```python
from build123d import *

# Parameters (mm, degrees)
BOSS_EXTRU_1_DEPTH      = 10
BOSS_EXTRU_2_DEPTH      = 48
BOSS_EXTRU_3_DEPTH      = 2
CHANFREIN1_SIZE         = 6
ENL_V_MAT_EXTRU_1_REACH = 148.244
ESQUISSE5_R             = 1.75
ESQUISSE6_R             = 3.5
ENL_V_MAT_EXTRU_2_DEPTH = 4
CHANFREIN2_SIZE         = 7.5
ESQUISSE7_R             = 1.25
ENL_V_MAT_EXTRU_3_DEPTH = 10


with BuildPart() as part:
    # Esquisse1 → Boss.-Extru.1 (new body)
    with BuildSketch(Plane.XY):
        with BuildLine():
            Line((-40.181760398, -97.007350914), (-47.835429046, -115.484941564))
            ThreePointArc((-47.835429046, -115.484941564), (-24.386290252, -122.59816005), (0, -125))
            Line((0, -125), (0, -105))
            ThreePointArc((0, -105), (-20.484483812, -102.982454442), (-40.181760398, -97.007350914))
        make_face()
    extrude(amount=BOSS_EXTRU_1_DEPTH)

    # Esquisse2 → Boss.-Extru.2 (add)
    with BuildSketch(Plane.XY.offset(10)):
        with BuildLine():
            Line((-32.925344295, -102.858746361), (-38.108037379, -119.049474955))
            ThreePointArc((-38.108037379, -119.049474955), (-24.386290252, -122.59816005), (-10.351025939, -124.570687812))
            Line((-10.351025939, -124.570687812), (-8.943286411, -107.62907427))
            ThreePointArc((-8.943286411, -107.62907427), (-21.069754778, -105.924810284), (-32.925344295, -102.858746361))
        make_face()
    extrude(amount=BOSS_EXTRU_2_DEPTH)

    # Esquisse4 → Boss.-Extru.3 (add)
    with BuildSketch(Plane.XY.offset(58)):
        with BuildLine():
            Line((-39.413172773, -123.12671677), (-10.705530953, -128.837021766))
            Line((-10.705530953, -128.837021766), (-8.943286411, -107.62907427))
            ThreePointArc((-8.943286411, -107.62907427), (-21.069754778, -105.924810284), (-32.925344295, -102.858746361))
            Line((-32.925344295, -102.858746361), (-39.413172773, -123.12671677))
        make_face()
    extrude(amount=BOSS_EXTRU_3_DEPTH)

    # Chanfrein1
    # the kernel refuses this chamfer: 6 mm, written as the material it adds along each edge
    with BuildSketch(Plane(origin=(0, 0, 58), x_dir=(-0.3048642990280114, -0.9523957996432781, 0), z_dir=(-0.9523957996432781, 0.3048642990280114, 0))) as chanfrein1_piece_1_section:
        Polygon((125 + CHANFREIN1_SIZE, 0), (125, -CHANFREIN1_SIZE), (125, 0), align=None)
    chanfrein1_piece_1 = revolve(axis=Axis((0, 0, 58), (0, 0, 1)), revolution_arc=13, mode=Mode.PRIVATE)
    chanfrein1_piece_1 = split(chanfrein1_piece_1, bisect_by=Plane(origin=(-25.059351863, -125.981869268, 58), z_dir=(0.19509032201612828, 0.9807852804032304, 0)), keep=Keep.TOP, mode=Mode.PRIVATE)
    add(chanfrein1_piece_1)

    # Esquisse5 → Enlèv. mat.-Extru.1 (cut, up to next)
    with BuildSketch(Plane.XY.offset(10), mode=Mode.PRIVATE) as enl_v_mat_extru_1_sk1:
        with Locations((-4.765565521, -114.901215769)):
            Circle(ESQUISSE5_R)
    enl_v_mat_extru_1_tool1 = extrude(enl_v_mat_extru_1_sk1.sketch, amount=-ENL_V_MAT_EXTRU_1_REACH, mode=Mode.PRIVATE) & part.part
    # Esquisse5 → Enlèv. mat.-Extru.1 (cut, up to next)
    with BuildSketch(Plane.XY.offset(10), mode=Mode.PRIVATE) as enl_v_mat_extru_1_sk2:
        with Locations((-39.567983188, -107.978584481)):
            Circle(ESQUISSE5_R)
    enl_v_mat_extru_1_tool2 = extrude(enl_v_mat_extru_1_sk2.sketch, amount=-ENL_V_MAT_EXTRU_1_REACH, mode=Mode.PRIVATE) & part.part
    add(enl_v_mat_extru_1_tool1.solids().sort_by_distance((-4.765566, -114.901216, 10))[0], mode=Mode.SUBTRACT)
    add(enl_v_mat_extru_1_tool2.solids().sort_by_distance((-39.567983, -107.978584, 10))[0], mode=Mode.SUBTRACT)

    # Esquisse6 → Enlèv. mat.-Extru.2 (cut)
    with BuildSketch(Plane.XY.offset(10)):
        with Locations((-39.567983188, -107.978584481)):
            Circle(ESQUISSE6_R)
        with Locations((-4.765565521, -114.901215769)):
            Circle(ESQUISSE6_R)
    extrude(amount=-ENL_V_MAT_EXTRU_2_DEPTH, mode=Mode.SUBTRACT)

    # Chanfrein2
    # the kernel refuses this chamfer: 7.5 mm, written as the material it takes off along each edge
    with BuildSketch(Plane(origin=(-8.943286411, -107.62907427, 10), x_dir=(-0.08280820751335238, -0.996565502497666, 0), z_dir=(0, 0, 1)), Plane(origin=(-32.925344295, -102.858746361, 80.019854797), x_dir=(-0.3048642990290983, -0.9523957996429303, 0), z_dir=(0, 0, -1))) as chanfrein2_piece_1:
        with BuildLine():
            Line((CHANFREIN2_SIZE, 0), (-0.280634385, -7.780634385))
            ThreePointArc((-0.280634385, -7.780634385), (-0.074202159, -4.002769088), (0, 0))
            Line((0, 0), (CHANFREIN2_SIZE, 0))
        make_face()
    extrude(amount=70.019854797, mode=Mode.SUBTRACT)

    # Esquisse7 → Enlèv. mat.-Extru.3 (cut)
    with BuildSketch(Plane.XY.offset(60)):
        with Locations((-30.083912118, -112.798307752)):
            Circle(ESQUISSE7_R)
        with Locations((-15.372132912, -115.724662582)):
            Circle(ESQUISSE7_R)
    extrude(amount=-ENL_V_MAT_EXTRU_3_DEPTH, mode=Mode.SUBTRACT)


solid = part.part
```
Work out the finished part from the listing and answer in its coordinate system (mm). A direction names the side the tool comes from. Give positions to 0.01 mm unless a question says otherwise; leave off trailing zeros. Loops run counter-clockwise (first coordinate to the right, second up) from the corner with the lowest first, then second, coordinate; pieces in that order, holes last. Notation, with made-up numbers: (69, -12.75) - (121, -12.75) arc R20 ccw to (121, 20.25) - close; hole circle Ø10 at (6, 81). An arc over 180 degrees is marked (long way). One line per question, with ' | ' between items.
(1) Each of these flat-tipped pins is pushed along its axis until it touches: pin 1 Ø10 at (x, z) = (-28, 18) entering from +Y; pin 2 Ø8 at (x, y) = (-4.77, -114.9) entering from +Z; pin 3 Ø5 at (x, z) = (-11, 27) entering from -Y; pin 4 Ø4 at (x, y) = (-15.37, -115.72) entering from +Z. Where does it stop, or does it pass through?
Recorded:
pin 1: stops at y = -104.96 | pin 2: stops at z = 10 | pin 3: stops at y = -124.57 | pin 4: stops at z = 60
(2) A tool of negligible diameter and unlimited length cuts with its end or side. For faces 1 (the face through (-13.07, -110.96, 34.65)), 2 (the face through (-30.39, -107.52, 35.35)), 3 (the face through (-15.643, -116.945, 55.07)), from which of +Z, -Z, +X, -X, +Y, -Y can it reach the whole face along a straight path? Write none if from no direction.
Recorded:
face 1: +Z, +X, +Y | face 2: +Z, -X, +Y | face 3: +Z
(3) Straight lines are drawn through the part: probe 1 along Z at (x, y) = (-39, -99.5); probe 2 along Y at (x, z) = (-32.5, 56); probe 3 along X at (y, z) = (-116.5, 56). For each, find the intervals that lie inside material, in ascending order.
Recorded:
probe 1: z = 0 to 10 | probe 2: y = -124.5 to -108.61 | probe 3: x = -37.29 to -16.35, -14.39 to -9.68
(4) The part is cut by section B-B (z = 41). Write down the section's boundary in (x, y).
Recorded:
outline: (-38.11, -119.05) arc R125 ccw to (-10.35, -124.57) - (-9.56, -115.1) - (-16.67, -106.71) arc R108 cw to (-25.43, -104.96) - (-35.21, -110) - close
(5) The part is cut by section A-A (z = 53). Write down the section's boundary in (x, y), then the cut area to 3 significant figures.
Recorded:
outline: (-38.41, -120) arc R126 ccw to (-10.43, -125.57) - (-9.56, -115.1) - (-16.67, -106.71) arc R108 cw to (-25.43, -104.96) - (-35.21, -110) - close; hole circle Ø2.5 at (-30.08, -112.8); hole circle Ø2.5 at (-15.37, -115.72) | area: 410 mm²
(6) The mould has two halves that part along X. Classify faces 4 (the face through (-15, -116, 50)), 5 (the face through (-24, -114, 0)), 6 (the face through (-43.955, -106.117, 4.93)): +X half, -X half, draft (parallel to the pull), parting line (faces both ways), or undercut.
Recorded:
face 4: undercut | face 5: draft | face 6: -X half
(7) The part is cut by section D-D (z = 4.5). Write down the section's boundary in (x, y).
Recorded:
outline: (-47.84, -115.48) arc R125 ccw to (0, -125) - (0, -105) arc R105 cw to (-40.18, -97.01) - close; hole circle Ø3.5 at (-39.57, -107.98); hole circle Ø3.5 at (-4.77, -114.9)
(8) The part is cut by section C-C (y = -103). Write down the section's boundary in (x, z).
Recorded:
outline: (-42.66, 0) - (-20.4, 0) - (-20.4, 10) - (-42.66, 10) - close
